Read the model definition and answer for the solid it produces. Units are mm, in the model's axes. Round coordinates to 2 decimals unless told otherwise and drop trailing zeros. Order: outer loops, then holes, each group sorted by start corner. A loop starts at its lowest first (then second) coordinate and runs counter-clockwise, first axis right, second up. Notation, with made-up numbers: (-33.5, -6.5) - (-8.5, -6.5) arc R30 cw to (-8.5, 15.5) - close; hole circle Ø2 at (82, 68). An arc over 180 degrees is marked (long way). Put each result on its own line as item: value. Start each with the question number.
Q1. For a pull along Z with two mould halves and no side action, classify faces 1 (the face through (96, 2, 0)), 2 (the face through (96, 0, -79)), 3 (the face through (96.198, 2.535, -101.415)), 4 (the face through (96, 2, -155)) as pulls with the +Z half, pulls with the -Z half, needs draft (parallel to the pull), parting line crosses it, or undercut.
Q2. Section B-B on z = -91.5 is taken. Give the vertices of the cut face in (x, y), then the cut area to 3 significant figures.
Q3. Find the intervals of material crossed by line 1 along X through (y, z) = (3.05, -150.5); line 2 along Z through (x, y) = (68, 3.6); line 3 along Z through (x, y) = (44, 3.1), in increasing order. Write a range as from..to.
Q4. Section C-C on y = 1.6 is taken. State how many separate pieces and enclosed holes the cut face has, then the cut area to 3 significant figures.
Q5. Each of these flat-tipped pins is pushed along its axis until it touches: pin 1 Ø5 at (x, z) = (44, -26.5) entering from -Y; pin 2 Ø2.5 at (x, z) = (107.5, -101.5) entering from -Y. Where does it stop, or does it pass through?
Q6. Section A-A on x = 80 is taken. Give the vertices of the cut face in (y, z), then the cut area to 3 significant figures.
from build123d import *

# Parameters (mm, degrees)
SKETCH1_W           = 194
SKETCH1_H           = 155
BOSS_EXTRUDE1_DEPTH = 5
SKETCH2_R           = 2
CUT_EXTRUDE1_DEPTH  = 6
SKETCH3_R           = 10
SKETCH3_R_2         = 1.5
CUT_EXTRUDE2_DEPTH  = 6
SKETCH4_R           = 2.25
CUT_EXTRUDE3_DEPTH  = 6
SKETCH5_R           = 1.5
CUT_EXTRUDE4_DEPTH  = 6
SKETCH6_R           = 1.5
CUT_EXTRUDE5_DEPTH  = 6


with BuildPart() as part:
    # Sketch1 → Boss-Extrude1 (new body)
    with BuildSketch(Plane(origin=(0, 0, 0), x_dir=(1, 0, 0), z_dir=(0, 1, 0))):
        with Locations((97, 77.5)):
            Rectangle(SKETCH1_W, SKETCH1_H)
    extrude(amount=BOSS_EXTRUDE1_DEPTH)

    # Sketch2 → Cut-Extrude1 (cut, through all)
    with BuildSketch(Plane(origin=(0, 5, 0), x_dir=(1, 0, 0), z_dir=(0, 1, 0))):
        with Locations((68, 121)):
            Circle(SKETCH2_R)
        with Locations((127, 121)):
            Circle(SKETCH2_R)
        with Locations((68, 62)):
            Circle(SKETCH2_R)
        with Locations((127, 62)):
            Circle(SKETCH2_R)
    extrude(amount=-CUT_EXTRUDE1_DEPTH, mode=Mode.SUBTRACT)

    # Sketch3 → Cut-Extrude2 (cut, through all)
    with BuildSketch(Plane(origin=(0, 5, 0), x_dir=(1, 0, 0), z_dir=(0, 1, 0))):
        with Locations((97.5, 91.5)):
            Circle(SKETCH3_R)
        with Locations((107.5, 101.5)):
            Circle(SKETCH3_R_2)
        with Locations((107.5, 81.5)):
            Circle(SKETCH3_R_2)
        with Locations((87.5, 81.5)):
            Circle(SKETCH3_R_2)
        with Locations((87.5, 101.5)):
            Circle(SKETCH3_R_2)
    extrude(amount=-CUT_EXTRUDE2_DEPTH, mode=Mode.SUBTRACT)

    # Sketch4 → Cut-Extrude3 (cut, through all)
    with BuildSketch(Plane(origin=(0, 0, 0), x_dir=(-1, 0, 0), z_dir=(0, -1, 0))):
        with Locations((-80, 6.896410277)):
            Circle(SKETCH4_R)
        with Locations((-105, 6.896410277)):
            Circle(SKETCH4_R)
        with Locations((-80, 36.396410277)):
            Circle(SKETCH4_R)
        with Locations((-105, 36.396410277)):
            Circle(SKETCH4_R)
    extrude(amount=-CUT_EXTRUDE3_DEPTH, mode=Mode.SUBTRACT)

    # Sketch5 → Cut-Extrude4 (cut, through all)
    with BuildSketch(Plane(origin=(0, 5, 0), x_dir=(1, 0, 0), z_dir=(0, 1, 0))):
        with Locations((10, 4.5)):
            Circle(SKETCH5_R)
        with Locations((44, 4.5)):
            Circle(SKETCH5_R)
        with Locations((44, 26.5)):
            Circle(SKETCH5_R)
        with Locations((10, 26.5)):
            Circle(SKETCH5_R)
        with Locations((150, 4.5)):
            Circle(SKETCH5_R)
        with Locations((150, 26.5)):
            Circle(SKETCH5_R)
        with Locations((184, 26.5)):
            Circle(SKETCH5_R)
        with Locations((184, 4.5)):
            Circle(SKETCH5_R)
        with Locations((150, 128.5)):
            Circle(SKETCH5_R)
        with Locations((150, 150.5)):
            Circle(SKETCH5_R)
        with Locations((184, 150.5)):
            Circle(SKETCH5_R)
        with Locations((184, 128.5)):
            Circle(SKETCH5_R)
        with Locations((10, 128.5)):
            Circle(SKETCH5_R)
        with Locations((10, 150.5)):
            Circle(SKETCH5_R)
        with Locations((44, 150.5)):
            Circle(SKETCH5_R)
        with Locations((44, 128.5)):
            Circle(SKETCH5_R)
    extrude(amount=-CUT_EXTRUDE4_DEPTH, mode=Mode.SUBTRACT)

    # Sketch6 → Cut-Extrude5 (cut, through all)
    with BuildSketch(Plane(origin=(0, 5, 0), x_dir=(1, 0, 0), z_dir=(0, 1, 0))):
        with Locations((5, 121.5)):
            Circle(SKETCH6_R)
        with Locations((60, 121.5)):
            Circle(SKETCH6_R)
        with Locations((5, 40.5)):
            Circle(SKETCH6_R)
        with Locations((60, 40.5)):
            Circle(SKETCH6_R)
    extrude(amount=-CUT_EXTRUDE5_DEPTH, mode=Mode.SUBTRACT)


solid = part.part
Findings:
1. face 1: pulls with the +Z half
1. face 2: needs draft
1. face 3: undercut
1. face 4: pulls with the -Z half
2. outline: (0, 0) - (87.5, 0) - (87.5, 5) - (0, 5) - close; (107.5, 0) - (194, 0) - (194, 5) - (107.5, 5) - close
2. area: 870 mm2
3. line 1: 0..8.5, 11.5..42.5, 45.5..148.5, 151.5..182.5, 185.5..194
3. line 2: -155..-123, -119..-64, -60..0
3. line 3: -155..-152, -149..-130, -127..-28, -25..-6, -3..0
4. separate pieces: 1
4. enclosed holes: 33
4. area: 29,500 mm2
5. pin 1: y = 0
5. pin 2: through
6. outline: (0, -155) - (5, -155) - (5, -38.65) - (0, -38.65) - close; (0, -34.15) - (5, -34.15) - (5, -9.15) - (0, -9.15) - close; (0, -4.65) - (5, -4.65) - (5, 0) - (0, 0) - close
6. area: 730 mm2
